Check sheet for the modelled part. Datum: model origin and axes. Units: mm. A direction names the side the tool comes from. Coordinates: 2 decimals unless noted, no trailing zeros. Write each loop counter-clockwise with the first axis right and the second up, starting at its lowest first coordinate (ties: lowest second). Pieces come first, ordered by that corner, then holes. Notation, with made-up numbers: (3, 14.25) -> (44, 14.25) arc R34 cw to (44, 46.25) -> close; hole circle Ø1 at (59.5, 18). An arc over 180 degrees is marked (long way). Put each result on its own line as item: value.
```python
from build123d import *
from build123d import SkipClean  # not in build123d's __all__

# Parameters (mm, degrees)
F0_W      = 101
F0_H      = 30
F1_DEPTH  = 18
F2_R      = 12
F3_DEPTH  = 8
F4_R      = 8
F5_DEPTH  = 38.001
F6_W      = 43
F6_H      = 14
F7_DEPTH  = 36.001
F9_DEPTH  = 16
F8_R      = 9
F10_DEPTH = 10
F12_DEPTH = 3
F13_R     = 8
F14_DEPTH = 22
F16_DEPTH = 7


# Not quite as in the source:
# - after a boolean that leaves OpenCascade's solid faulty, fix() repairs it


with BuildPart() as f1:
    # F0 (on Right) → F1 (new body, symmetric)
    with BuildSketch(Plane.YZ):
        Rectangle(F0_W, F0_H)
    extrude(amount=F1_DEPTH, both=True)

    # F2 (on face) → F3 (join)
    with BuildSketch(Plane.XY.offset(15)):
        with Locations((0, 32.5)):
            Circle(F2_R)
    extrude(amount=F3_DEPTH)

    # F4 (on face) → F5 (cut, through all)
    with BuildSketch(Plane.XY.offset(23)):
        with Locations((0, 32.5)):
            Circle(F4_R)
    extrude(amount=-F5_DEPTH, mode=Mode.SUBTRACT)

    # F6 (on face) → F7 (cut, through all)
    with BuildSketch(Plane.YZ.offset(18)):
        with Locations((-29, 8)):
            Rectangle(F6_W, F6_H)
    extrude(amount=-F7_DEPTH, mode=Mode.SUBTRACT)

    # F8 (on face) → F9 (join)
    with BuildSketch(Plane.XY.offset(1)):
        with BuildLine():
            Line((-9, -50.5), (9, -50.5))
            ThreePointArc((9, -50.5), (0, -41.5), (-9, -50.5))
        make_face()
        with BuildLine():
            ThreePointArc((-9, -50.5), (0, -59.5), (9, -50.5))
            Line((9, -50.5), (-9, -50.5))
        make_face()
    extrude(amount=-F9_DEPTH)

    # F8 (on face) → F10 (join)
    with BuildSketch(Plane.XY.offset(1)):
        with Locations((0, -50.5)):
            Circle(F8_R)
    with SkipClean():  # cleaning this boolean's faces spoils the solid; the shape is the same uncleaned
        extrude(amount=F10_DEPTH)

    # F11 (on Right) → F12 (join, symmetric)
    with BuildSketch(Plane.YZ):
        Polygon((-7.5, 1), (-7.5, 15), (-32.5, 1), align=None)
    extrude(amount=F12_DEPTH, both=True)

    add(f1.part.fix(), mode=Mode.REPLACE)

    # F13 (on face) → F14 (cut)
    with BuildSketch(Plane(origin=(0, 0, -15), x_dir=(1, 0, 0), z_dir=(0, 0, -1))):
        with BuildLine():
            Line((-14, 2.5), (-14, -32.5))
            ThreePointArc((-14, -32.5), (0, -46.5), (14, -32.5))
            Line((14, -32.5), (14, 2.5))
            Line((14, 2.5), (-14, 2.5))
        make_face()
        with Locations((0, -32.5)):
            Circle(F13_R, mode=Mode.SUBTRACT)
    extrude(amount=-F14_DEPTH, mode=Mode.SUBTRACT)

    # F15 (on face) → F16 (cut)
    with BuildSketch(Plane(origin=(0, 0, -15), x_dir=(1, 0, 0), z_dir=(0, 0, -1))):
        with BuildLine():
            Line((9, 2.5), (9, 27.5))
            ThreePointArc((9, 27.5), (0, 36.5), (-9, 27.5))
            Line((-9, 27.5), (-9, 2.5))
            Line((-9, 2.5), (9, 2.5))
        make_face()
    extrude(amount=-F16_DEPTH, mode=Mode.SUBTRACT)


solid = f1.part
```
Q1. Cross-section at B-B (z = 6). Record the cut outline in (x, y), plus the area to 3 significant figures.
Recorded:
outline: (-18, -7.5) -> (-3, -7.5) -> (-3, -23.57) -> (3, -23.57) -> (3, -7.5) -> (18, -7.5) -> (18, 50.5) -> (-18, 50.5) -> close; circle Ø18 at (0, -50.5); hole (-14, -2.5) -> (14, -2.5) -> (14, 32.5) arc R14 ccw to (-14, 32.5) -> close
area: 1,150 mm2
Q2. Cross-section at A-A (x = 0). Record the cut outline in (y, z), plus the area to 3 significant figures.
Recorded:
outline: (-59.5, -15) -> (-36.5, -15) -> (-36.5, -8) -> (-2.5, -8) -> (-2.5, 7) -> (24.5, 7) -> (24.5, 23) -> (20.5, 23) -> (20.5, 15) -> (-7.5, 15) -> (-32.5, 1) -> (-41.5, 1) -> (-41.5, 11) -> (-59.5, 11) -> close; (40.5, 7) -> (46.5, 7) -> (46.5, -15) -> (50.5, -15) -> (50.5, 15) -> (44.5, 15) -> (44.5, 23) -> (40.5, 23) -> close
area: 1,550 mm2
Q3. Cross-section at C-C (z = -0.5). Record the cut outline in (x, y).
Recorded:
outline: (-18, -50.5) -> (-9, -50.5) arc R9 ccw to (9, -50.5) -> (18, -50.5) -> (18, 50.5) -> (-18, 50.5) -> close; hole (-14, -2.5) -> (14, -2.5) -> (14, 32.5) arc R14 ccw to (-14, 32.5) -> close
Q4. Mould release check, pull along Y, two halves, no side actions. Record for faces 1 (the flat face through (0, 50.5, 0)), 2 (the flat face through (0, 16, 7)), 3 (the flat face through (-13, -50.5, -7)), 4 (the flat face through (0, -50, 11)): released by +Y, released by -Y, zero draft, split by the parting line, or undercut.
Recorded:
face 1: released by +Y
face 2: undercut
face 3: released by -Y
face 4: zero draft
Q5. Depth check by flat-ended pin: P1, Ø11, axis at x = 5, y = -26, coming from the +Z side; P2, Ø20, axis at x = -2, y = -24, coming from the -Z side; P3, Ø6, axis at x = -10, z = 14.5, coming from the -Y side; P4, Ø3, axis at x = 0.5, z = 14, coming from the -Y side. Enter the tip coordinate at first touch or a pass-through.
Recorded:
P1: stops at z = 7.51
P2: stops at z = -15
P3: stops at y = -7.5
P4: stops at y = -11.96
Q6. Material ranges on line 1 along X through (y, z) = (32, 10); line 2 along Y through (x, z) = (0, 16); line 3 along X through (y, z) = (-22, -12), recorded low to high.
Recorded:
line 1: x = -18 to -7.98, 7.98 to 18
line 2: y = 20.5 to 24.5, 40.5 to 44.5
line 3: x = -18 to -9, 9 to 18
Q7. Tool access check on faces 5 (the flat face through (11, -7.5, 8)), 6 (the cylindrical face through (6.45, 42.62, 18.94)), 7 (the flat face through (0, -20, 8)), 8 (the flat face through (14, 15, -4)), 9 (the flat face through (-3, -15, 5)). Record the directions out of +Z, -Z, +X, -X, +Y, -Y that give a thin tool (end or side, any length) a straight path to the whole face; none if there is none.
Recorded:
face 5: +Z, +X
face 6: +Z
face 7: +Z, +X, -X
face 8: -Z
face 9: +Z, -X
Q8. Cross-section at D-D (y = -11). Record the cut outline in (x, z), plus the area to 3 significant figures.
Recorded:
outline: (-18, -15) -> (-9, -15) -> (-9, -8) -> (9, -8) -> (9, -15) -> (18, -15) -> (18, 1) -> (3, 1) -> (3, 13.04) -> (-3, 13.04) -> (-3, 1) -> (-18, 1) -> close
area: 522 mm2
